```python
from build123d import *

# Parameters (mm, degrees)
CHAMFER_1_SIZE                       = 1
CHAMFER_2_SIZE                       = 1
FILLET_1_R                           = 0.2
SKETCH_5_R                           = 1.2
CUT_EXTRUDE_2_DEPTH                  = 2
CHAMFER_3_SIZE                       = 0.5
PATTERN_CIRCULAR_1_COUNT             = 2
CHAMFER_3_OF_PATTERN_CIRCULAR_1_SIZE = 0.5


with BuildPart() as part:
    # 스케치3 → 회전2 (revolve)
    with BuildSketch(Plane(origin=(0, 0, 0), x_dir=(1, 0, 0), z_dir=(0, 1, 0)), mode=Mode.PRIVATE) as revolve_2_sk:
        Polygon((11.1, 0), (11.1, -2.5), (8.6, -2.5), (8.6, -4.3), (9.5, -5.1), (9.5, -8.2), (9.4, -8.2), (9.4, -8.4), (9.5, -8.4), (9.5, -11.1), (10.05, -11.65), (10.05, -16.25), (9.5, -16.8), (9.5, -19.8), (2.9, -19.8), (2.9, -11.8), (4.4, -11.8), (4.4, -10), (3.4, -10), (3.4, -8.5), (6.1, -7.77653718), (6.1, 0), align=None)
    revolve(revolve_2_sk.sketch.rotate(Axis((0, 0, 0), (0, 0, 1)), 180), axis=Axis((0, 0, 0), (0, 0, 1)))

    # 모따기1
    chamfer_1_edges = [part.edges().sort_by_distance(p)[0] for p in [
        (6.1, 0, 0),
        (9.5, 0, 19.8),
    ]]
    chamfer(chamfer_1_edges, length=CHAMFER_1_SIZE)

    # 모따기2
    chamfer_2_edges = [part.edges().sort_by_distance(p)[0] for p in [
        (11.1, 0, 0),
    ]]
    chamfer(chamfer_2_edges, length=CHAMFER_2_SIZE)

    # 필렛1
    fillet_1_edges = [part.edges().sort_by_distance(p)[0] for p in [
        (11.1, 0, 2.5),
    ]]
    fillet(fillet_1_edges, radius=FILLET_1_R)

    # 스케치5 → 컷-돌출2 (cut)
    with BuildSketch(Plane(origin=(0, 10.05, 0), x_dir=(1, 0, 0), z_dir=(0, 1, 0))):
        with Locations(Location((0, -14, 0), (0, 0, 270))):
            Circle(SKETCH_5_R)
    cut_extrude_2 = extrude(amount=-CUT_EXTRUDE_2_DEPTH, mode=Mode.SUBTRACT)

    # 모따기3
    chamfer_3_edges = [part.edges().sort_by_distance(p)[0] for p in [
        (0, 8.05, 12.8),
    ]]
    chamfer(chamfer_3_edges, length=CHAMFER_3_SIZE)

    # 원형 패턴1: 컷-돌출2 ×2 about axis
    pattern_circular_1_axis = Axis((0, 0, 0), (0, 0, -1))
    for i in range(1, PATTERN_CIRCULAR_1_COUNT):
        add(cut_extrude_2.rotate(pattern_circular_1_axis, i * 360 / PATTERN_CIRCULAR_1_COUNT), mode=Mode.SUBTRACT)

    # 모따기3 of 원형 패턴1
    chamfer_3_of_pattern_circular_1_edges = [part.edges().sort_by_distance(p)[0] for p in [
        (0, -8.05, 12.8),
    ]]
    chamfer(chamfer_3_of_pattern_circular_1_edges, length=CHAMFER_3_OF_PATTERN_CIRCULAR_1_SIZE)


solid = part.part
```
Could you check a few things on this model? Use its own coordinates, in mm. A direction names the side the tool comes from. Give positions to 0.01 mm unless a question says otherwise; leave off trailing zeros. Loops run counter-clockwise (first coordinate to the right, second up) from the corner with the lowest first, then second, coordinate; pieces in that order, holes last. Notation, with made-up numbers: (80, -23) -> (125, -23) arc R19 ccw to (125, 3) -> close; hole circle Ø11 at (20, 69.25). An arc over 180 degrees is marked (long way). Put each result on its own line as item: value.
(1) Please list where these lines run through material, in increasing order: probe 1 along Z at (x, y) = (0, 9.2); probe 2 along Z at (x, y) = (0, 9.55); probe 3 along Y at (x, z) = (1.75, 3.75). Write a range as [from, to].
Computed:
probe 1: [0, 2.5], [4.83, 12.8], [15.2, 19.1]
probe 2: [0, 2.5], [11.15, 12.8], [15.2, 16.75]
probe 3: [-8.42, -5.84], [5.84, 8.42]
(2) Imagine slicing it at B-B on z = 3. Write out the boundary of the cut face in (x, y), plus the area to 3 significant figures.
Computed:
outline: circle Ø17.2 at (0, 0); hole circle Ø12.2 at (0, 0)
area: 115 mm^2
(3) Imagine slicing it at A-A on z = 14. Write out the boundary of the cut face in (x, y), plus the area to 3 significant figures.
Computed:
outline: (-1.2, -9.98) -> (-1.2, -8.55) -> (-0.7, -8.05) -> (0.7, -8.05) -> (1.2, -8.55) -> (1.2, -9.98) arc R10.05 ccw to (1.2, 9.98) -> (1.2, 8.55) -> (0.7, 8.05) -> (-0.7, 8.05) -> (-1.2, 8.55) -> (-1.2, 9.98) arc R10.05 ccw to start; hole circle Ø5.8 at (0, 0)
area: 282 mm^2
(4) Thinking about a two-plate mould opening in Y: for faces 1 (the face through (0, 8.05, 14)), 2 (the face through (-0.05, -9.31, 12.8)), 3 (the face through (0.74, 3.32, 9.24)), which applies, pulls with the +Y half, pulls with the -Y half, needs draft (parallel to the pull), parting line crosses it, or undercut?
Computed:
face 1: pulls with the +Y half
face 2: needs draft
face 3: undercut
(5) Imagine slicing it at C-C on z = 17.25. Write out the boundary of the cut face in (x, y), plus the area to 3 significant figures.
Computed:
outline: circle Ø19 at (0, 0); hole circle Ø5.8 at (0, 0)
area: 257 mm^2
(6) For faces 4 (the face through (-1, -9, 2.5)), 5 (the face through (0.05, 9.31, 12.8)), 6 (the face through (6.094, -0.268, 4.341)), 7 (the face through (10.04, -0.44, 13.98)), 8 (the face through (0, -8.05, 14)), which set-ups out of +Z, -Z, +X, -X, +Y, -Y let a thin tool reach every point of the face, with its end or its side?
Computed:
face 4: none
face 5: +Y
face 6: -Z
face 7: +Z
face 8: -Y
(7) I'm going to push flat-ended pins straight in: pin 1 Ø2 at (x, z) = (0, 14) entering from -Y; pin 2 Ø1.5 at (y, z) = (5, 4.5) entering from +X; pin 3 Ø1.1 at (x, z) = (0, 14) entering from -Y; pin 4 Ø2.5 at (x, y) = (0.5, -0.5) entering from +Z. Where does each tip first touch, or does it pass through?
Computed:
pin 1: y = -8.35
pin 2: x = 8.34
pin 3: y = -8.05
pin 4: through
